```python
from build123d import *

# Parameters (mm, degrees)
F0_W     = 60
F0_H     = 40
F1_DEPTH = 10
F3_DEPTH = 20
F5_DEPTH = 25
F7_DEPTH = 10
F8_R     = 9.99999


# Not quite as in the source:
# - a fillet or chamfer is up to 0.001 mm smaller than in the source, because OpenCascade refuses the exact size


with BuildPart() as f1:
    # F0 (on Top) → F1 (new body)
    with BuildSketch(Plane.XY):
        with Locations((30, 20)):
            Rectangle(F0_W, F0_H)
    extrude(amount=F1_DEPTH)

    # F2 (on Front) → F3 (join)
    with BuildSketch(Plane.XZ):
        with BuildLine():
            Line((50, 20), (40, 20))
            ThreePointArc((40, 20), (20, 40), (0, 20))
            Line((0, 20), (0, 10))
            Line((0, 10), (60, 10))
            ThreePointArc((60, 10), (57.0710678119, 17.0710678119), (50, 20))
        make_face()
    extrude(amount=-F3_DEPTH)

    # F4 (on face) → F5 (cut)
    with BuildSketch(Plane.XZ):
        with BuildLine():
            ThreePointArc((30, 20), (12.928932207, 27.0710678307), (19.9999999466, 10))
            ThreePointArc((19.9999999466, 10), (27.071067793, 12.9289321693), (30, 20))
        make_face()
    extrude(amount=-F5_DEPTH, mode=Mode.SUBTRACT)

    # F6 (on face) → F7 (join)
    with BuildSketch(Plane(origin=(0, 40, 0), x_dir=(-1, 0, 0), z_dir=(0, 1, 0))):
        Polygon((-60, 30), (-60, 10), (-40, 10), (-40, 20), (-50, 20), (-50, 30), align=None)
    extrude(amount=-F7_DEPTH)

    # F8 (radius 10 in the source; OpenCascade refuses exactly that, so slightly less here)
    f8_edges = [f1.edges().sort_by_distance(p)[0] for p in [
        (50, 35, 20),
    ]]
    fillet(f8_edges, radius=F8_R)


solid = f1.part
```
The listing builds one solid part. Answer for the finished solid, in the listing's coordinates (mm). A direction names the side the tool comes from. Coordinates: 2 decimals unless noted, no trailing zeros. Loops run counter-clockwise (first coordinate to the right, second up) from the corner with the lowest first, then second, coordinate; pieces in that order, holes last. Notation, with made-up numbers: M -18.75,88.25 L 38.25,88.25 A21 ccw 38.25,115.25 Z; hole C -10,-7.75 d1. An arc over 180 degrees is marked long. Answer as a JSON object with one key per item and string values. Group by question number.
Item 1: Section B-B (x = 23) is taken. Write down the section's boundary in (y, z).
Item 2: Section A-A (y = 13.5) is taken. Write down the section's boundary in (x, z).
Item 3: Each of these flat-tipped pins is pushed along its axis until it touches: P1, Ø8, axis at y = 10.5, z = 19, coming from the +X side; P2, Ø4, axis at x = 10, z = 14, coming from the +Y side; P3, Ø5, axis at y = 27, z = 13.5, coming from the +X side (3 decimals); P4, Ø4, axis at x = 23, y = 12.5, coming from the +Z side (3 decimals). Where does it stop, or does it pass through?
Item 4: Section C-C (x = 36) is taken. Write down the section's boundary in (y, z), and give its area (3 significant figures).
Item 5: Which of the six approach directions +Z, -Z, +X, -X, +Y, -Y give full straight-line access (tool end or side, diameter ignored) to faces 1 (the face through (57.15, 9.86, 16.99)), 2 (the face through (40, 35, 15)), 3 (the face through (30, 20, 25))?
Item 6: Consider L1, parallel to Z at x = 20, y = 16; L2, parallel to Y at x = 31.5, z = 12; L3, parallel to Z at x = 51.5, y = 30.5. Determine where each line is inside the solid, lowest interval first.
Item 7: Section D-D (z = 34) is taken. Write down the section's boundary in (x, y), and give its area (3 significant figures).
Solved:
{
 "1": {"outline": "M 0,0 L 40,0 L 40,10 L 20,10 L 20,10.46 L 0,10.46 Z; M 0,29.54 L 20,29.54 L 20,39.77 L 0,39.77 Z"},
 "2": {"outline": "M 0,0 L 60,0 L 60,10 A10 ccw 50,20 L 40,20 A20 ccw 0,20 Z; hole C 20,20 d20"},
 "3": {"P1": "stops at x = 58.66", "P2": "stops at y = 20", "P3": "passes through", "P4": "stops at z = 39.975"},
 "4": {"outline": "M 0,0 L 40,0 L 40,10 L 20,10 L 20,32 L 0,32 Z", "area": "840 mm2"},
 "5": {"face 1": "+Z, +X, -Y", "face 2": "+Z, -X, +Y", "face 3": "+Z, +X, -X"},
 "6": {"L1": "z = 0 to 10, 30 to 40", "L2": "y = 0 to 20", "L3": "z = 0 to 30"},
 "7": {"outline": "M 5.72,0 L 34.28,0 L 34.28,20 L 5.72,20 Z", "area": "571 mm2"}
}
